Read the model definition and answer for the solid it produces. Units are mm, in the model's axes. Face numbers are marked on the shaded views. A direction names the side the tool comes from. Give positions to 0.01 mm unless a question says otherwise; leave off trailing zeros. Write each loop counter-clockwise with the first axis right and the second up, starting at its lowest first coordinate (ties: lowest second). Pieces come first, ordered by that corner, then holes. Notation, with made-up numbers: (73, -2.5) - (132, -2.5) arc R14 ccw to (132, 16.5) - close; hole circle Ø9 at (-7, 14.25). An arc over 180 degrees is marked (long way). Answer as CSV lines item,"result".
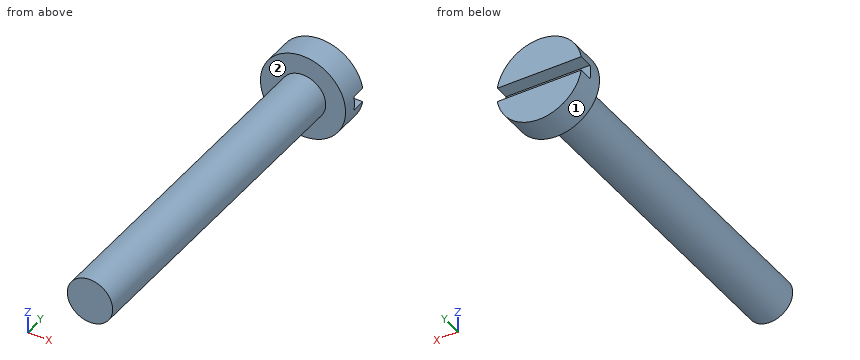
Autodesk Inventor part; units mm, degrees
ref_plane "YZ Plane" through (0, 0, 0) normal (1, 0, 0) x (0, 1, 0)
ref_plane "XZ Plane" through (0, 0, 0) normal (0, 1, 0) x (-1, 0, 0)
ref_plane "XY Plane" through (0, 0, 0) normal (0, 0, 1) x (1, 0, 0)
sketch "Sketch1" plane through (0, 0, 0) normal (0, 1, 0) x (-1, 0, 0)
  circle A0 centre (0, 0) radius 0.8
  dimension "d0" = 1.6
extrude "Extrusion1" add sketch "Sketch1" along normal blind 13
sketch "Sketch2" plane through (0, 13, 0) normal (0, 1, 0) x (1, 0, 0)
  circle A0 centre (0, 0) radius 0.8
  circle A1 centre (0, 0) radius 1.5
  dimension "d3" = 3
extrude "Extrusion2" add sketch "Sketch2" against normal blind 1
sketch "Sketch3" plane through (0, 13, 0) normal (0, 1, 0) x (1, 0, 0)
  line L0 (2, -0.25) -> (-2, -0.25)
  line L1 (-2, -0.25) -> (-2, 0.25)
  line L2 (-2, 0.25) -> (2, 0.25)
  line L3 (2, 0.25) -> (2, -0.25)
  line L4 (2, -0.25) -> (-2, 0.25) construction
  line L5 (-2, -0.25) -> (2, 0.25) construction
  point P0 (0, 0)
  dimension "d6" = 0.5
  dimension "d7" = 4
extrude "Extrusion3" cut sketch "Sketch3" against normal blind 0.5
properties part number "M1.6x0.35 Bolt" material "Aluminum 6061"
(1) A cutting plane is placed at D-D (x = 0). Write down the section's boundary in (y, z), and give its area (4 significant figures).
Worked out:
outline,"(0, -0.8) - (12, -0.8) - (12, -1.5) - (13, -1.5) - (13, -0.25) - (12.5, -0.25) - (12.5, 0.25) - (13, 0.25) - (13, 1.5) - (12, 1.5) - (12, 0.8) - (0, 0.8) - close"
area,"21.95 mm^2"
(2) For the marked faces 1 and 2, determine the directions among +Z, -Z, +X, -X, +Y, -Y from which every point of the face is accessible in a straight line to the end or side of a thin tool.
Worked out:
face 1,"+Y, -Y"
face 2,"-Y"
(3) A cutting plane is placed at C-C (y = 11.5). Write down the section's boundary in (x, z).
Worked out:
outline,"circle Ø1.6 at (0, 0)"
(4) A cutting plane is placed at A-A (x = 1.2). Write down the section's boundary in (y, z).
Worked out:
outline,"(12, -0.9) - (13, -0.9) - (13, -0.25) - (12.5, -0.25) - (12.5, 0.25) - (13, 0.25) - (13, 0.9) - (12, 0.9) - close"
(5) A cutting plane is placed at B-B (z = 0). Write down the section's boundary in (x, y), and give its area (3 significant figures).
Worked out:
outline,"(-1.5, 12) - (-0.8, 12) - (-0.8, 0) - (0.8, 0) - (0.8, 12) - (1.5, 12) - (1.5, 12.5) - (-1.5, 12.5) - close"
area,"20.7 mm^2"
(6) Find the intervals of material crossed by L1, parallel to Y at x = -0.4, z = 0.9; L2, parallel to X at y = 5, z = 0; L3, parallel to Z at x = -0.7, y = 7.75, in increasing order.
Worked out:
L1,"y = 12 to 13"
L2,"x = -0.8 to 0.8"
L3,"z = -0.39 to 0.39"
